```python
from build123d import *

# Parameters (mm, degrees)
F0_R     = 7.5
F1_DEPTH = 1
F2_R     = 4.942542
F3_DEPTH = 4
F4_R     = 7.5
F5_DEPTH = 1
F6_R     = 2.5
F7_DEPTH = 25


with BuildPart() as f1:
    # F0 (on Front) → F1 (new body)
    with BuildSketch(Plane.XZ):
        Circle(F0_R)
    extrude(amount=F1_DEPTH)

    # F2 (on face) → F3 (join)
    with BuildSketch(Plane.XZ.offset(1)):
        Circle(F2_R)
    extrude(amount=F3_DEPTH)

    # F4 (on face) → F5 (join)
    with BuildSketch(Plane.XZ.offset(5)):
        Circle(F4_R)
    extrude(amount=F5_DEPTH)

    # F6 (on face) → F7 (cut)
    with BuildSketch(Plane.XZ.offset(6)):
        Circle(F6_R)
    extrude(amount=-F7_DEPTH, mode=Mode.SUBTRACT)


solid = f1.part
```
Build history of the part. All positions in model axes, mm. A direction names the side the tool comes from. Give positions to 0.01 mm unless a question says otherwise; leave off trailing zeros. Loops run counter-clockwise (first coordinate to the right, second up) from the corner with the lowest first, then second, coordinate; pieces in that order, holes last. Notation, with made-up numbers: (5, -34.5) -> (35, -34.5) arc R24 cw to (35, 3.5) -> close; hole circle Ø5 at (87, -15.75). An arc over 180 degrees is marked (long way). One line per question, with ' | ' between items. Start each with the question number.
1) Cut at D-D (z = 3). Give the cut face in (x, y), plus the area to 3 significant figures.
2) Two-plate mould, pull along Y, no slides. Class faces 3 (the flat face through (2, -5, -5)), 4 (the flat face through (-2, -6, 2)), 5 (the cylindrical face through (-0.54, -3.04, -2.44)): released by +Y, released by -Y, zero draft, split by the parting line, or undercut.
3) Cut at A-A (z = 0). Give the cut face in (x, y).
4) Cut at C-C (y = -0.75). Give the cut face in (x, z).
5) 3-axis set-ups, long thin cutter, end or side, ignore diameter. For faces 1 (the flat face through (-2, 0, 2)), 2 (the flat face through (2, -1, -5)): which of +Z, -Z, +X, -X, +Y, -Y reach the whole face in a straight line?
6) Cut at B-B (x = 2.25). Give the cut face in (y, z).
7) Probe L1, parallel to Y at x = -1.5, z = 7.25; L2, parallel to Z at x = 0, y = -3.9; L3, parallel to X at y = -3.6, z = 1.25. List the from-to ranges inside material, lowest first.
8) Pin check, flat tips, straight feed: pin 1 (3 mm diameter, centred on x = -4.5, y = -4, fed in from -Z); pin 2 (1 mm diameter, centred on y = -3.5, z = 4, fed in from -X); pin 3 (2 mm diameter, centred on x = 5, y = -1.5, fed in from +Z). Stop position of each tip, or through.
Return value:
1) outline: (-6.87, -6) -> (6.87, -6) -> (6.87, -5) -> (3.93, -5) -> (3.93, -1) -> (6.87, -1) -> (6.87, 0) -> (-6.87, 0) -> (-6.87, -1) -> (-3.93, -1) -> (-3.93, -5) -> (-6.87, -5) -> close | area: 58.9 mm^2
2) face 3: undercut | face 4: released by -Y | face 5: zero draft
3) outline: (-7.5, -6) -> (-2.5, -6) -> (-2.5, 0) -> (-7.5, 0) -> (-7.5, -1) -> (-4.94, -1) -> (-4.94, -5) -> (-7.5, -5) -> close; (2.5, -6) -> (7.5, -6) -> (7.5, -5) -> (4.94, -5) -> (4.94, -1) -> (7.5, -1) -> (7.5, 0) -> (2.5, 0) -> close
4) outline: circle Ø15 at (0, 0); hole circle Ø5 at (0, 0)
5) face 1: +Z, -Z, +X, -X, +Y | face 2: none
6) outline: (-6, -7.15) -> (-5, -7.15) -> (-5, -4.4) -> (-1, -4.4) -> (-1, -7.15) -> (0, -7.15) -> (0, -1.09) -> (-6, -1.09) -> close; (-6, 1.09) -> (0, 1.09) -> (0, 7.15) -> (-1, 7.15) -> (-1, 4.4) -> (-5, 4.4) -> (-5, 7.15) -> (-6, 7.15) -> close
7) L1: -6 to -5, -1 to 0 | L2: -4.94 to -2.5, 2.5 to 4.94 | L3: -4.78 to -2.17, 2.17 to 4.78
8) pin 1: z = -6.69 | pin 2: x = -3.49 | pin 3: z = 6.26
